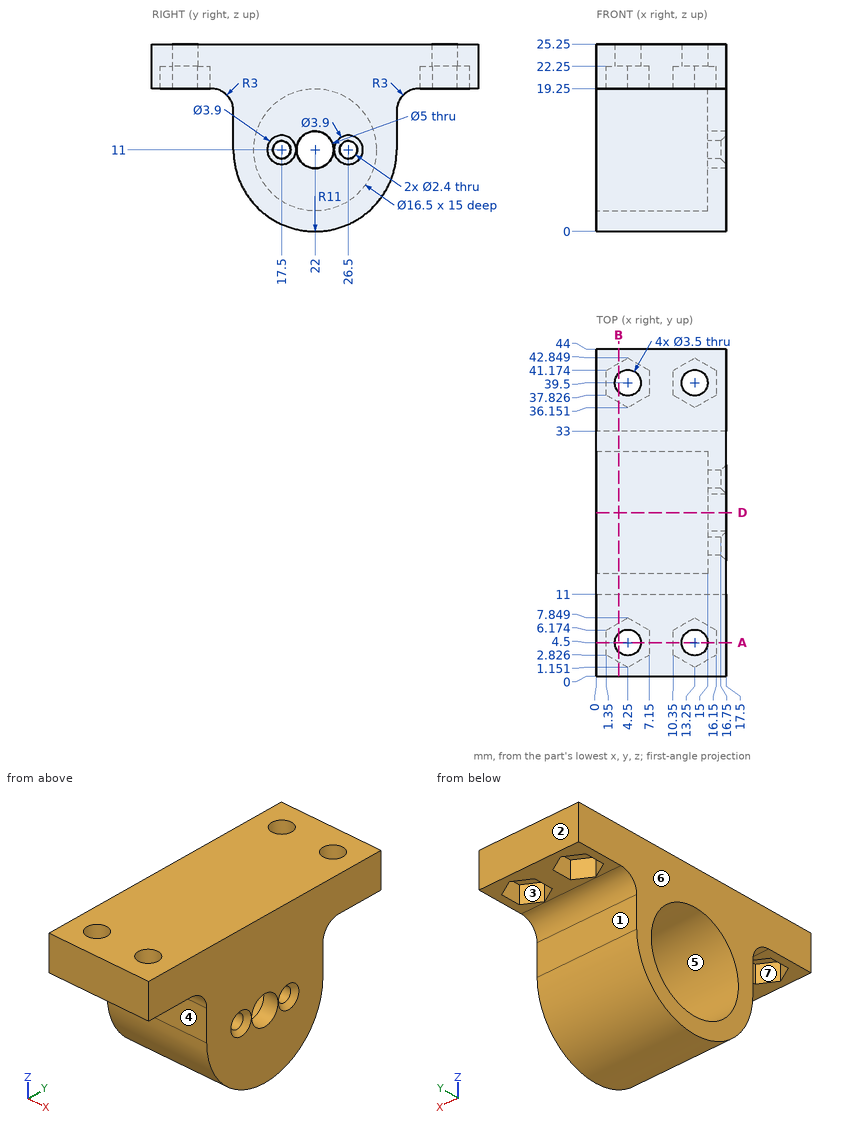
Drawing for the job (mm, zero at the part's lowest x, y, z). A direction names the side the tool comes from. Round coordinates to 2 decimals unless told otherwise and drop trailing zeros. Loops run counter-clockwise (first coordinate to the right, second up) from the corner with the lowest first, then second, coordinate; pieces in that order, holes last. Notation, with made-up numbers: (52, -26.75) - (111, -26.75) arc R16 cw to (111, -22.75) - close; hole circle Ø9 at (31.25, -28). An arc over 180 degrees is marked (long way). Return JSON: item names as keys, results as strings. Group by question number.
Q1. Band-saw the part on A-A on y = 4.5. Give the cut face in (x, z), plus the area to 3 significant figures.
Q2. Two-plate mould, pull along X, no slides. Class the marked faces 5, 6 and 7: +X half, -X half, draft (parallel to the pull), parting line (faces both ways), or undercut.
Q3. Drill centre lines: line 1 along Y through (x, z) = (15.55, 11); line 2 along X through (y, z) = (4.5, 23.55); line 3 along Y through (x, z) = (13, 23.5). Where is each one in solid material? Low to high. Write a range as [from, to].
Q4. Band-saw the part on D-D on y = 22. Give the cut face in (x, z).
Q5. Flat gauge pins, fed straight in: pin 1 Ø8 at (x, z) = (8, 13.5) entering from -Y; pin 2 Ø4 at (x, z) = (7.5, 14) entering from -Y; pin 3 Ø3 at (y, z) = (26.5, 11) entering from -X. Where does each tip first touch, or does it go through?
Q6. Tool access for the marked faces 1, 2, 3 and 4: list every direction of +Z, -Z, +X, -X, +Y, -Y with a clear straight run to the whole face (end or side of a thin tool).
Q7. Band-saw the part on B-B on x = 3. Give the number of separate pieces and of enclosed holes in the cut face.
Solutions:
{
 "1": {"outline": "(0, 19.25) - (1.35, 19.25) - (1.35, 22.25) - (2.5, 22.25) - (2.5, 25.25) - (0, 25.25) - close; (6, 22.25) - (7.15, 22.25) - (7.15, 19.25) - (10.35, 19.25) - (10.35, 22.25) - (11.5, 22.25) - (11.5, 25.25) - (6, 25.25) - close; (15, 22.25) - (16.15, 22.25) - (16.15, 19.25) - (17.5, 19.25) - (17.5, 25.25) - (15, 25.25) - close", "area": "49.2 mm^2"},
 "2": {"face 5": "draft", "face 6": "-X half", "face 7": "undercut"},
 "3": {"line 1": "y = [11, 16.3], [18.7, 19.5], [24.5, 25.3], [27.7, 33]", "line 2": "x = [0, 2.5], [6, 11.5], [15, 17.5]", "line 3": "y = [0, 2.77], [6.23, 37.77], [41.23, 44]"},
 "4": {"outline": "(0, 0) - (17.5, 0) - (17.5, 8.5) - (15, 8.5) - (15, 2.75) - (0, 2.75) - close; (0, 19.25) - (15, 19.25) - (15, 13.5) - (17.5, 13.5) - (17.5, 25.25) - (0, 25.25) - close"},
 "5": {"pin 1": "stops at y = 10.73", "pin 2": "stops at y = 11", "pin 3": "stops at x = 15"},
 "6": {"face 1": "-Z, +X, -X, +Y", "face 2": "+Z, -Z, +X, -X, +Y", "face 3": "-Z", "face 4": "-Z, +X, -X, -Y"},
 "7": {"separate pieces": "3", "enclosed holes": "1"}
}
